The listing builds one solid part. Answer for the finished solid, in the listing's coordinates (mm). A direction names the side the tool comes from. Round coordinates to 2 decimals unless told otherwise and drop trailing zeros. Order: outer loops, then holes, each group sorted by start corner. A loop starts at its lowest first (then second) coordinate and runs counter-clockwise, first axis right, second up. Notation, with made-up numbers: M 35,73.5 L 65,73.5 A17 ccw 65,100.5 Z; hole C -14,46 d10. An arc over 180 degrees is marked long. Put each result on its own line as item: value. Start each with the question number.
1. The mould has two halves that part along X. Classify faces 1 (the face through (39, 7.3, -1)), 2 (the face through (-73, 20, 7.5)), 3 (the face through (71.993, 19.748, -40.325)): +X half, -X half, draft (parallel to the pull), parting line (faces both ways), or undercut.
2. The part is cut by section A-A (x = -49). Give the vertices of the cut face in (y, z), then the cut area to 3 significant figures.
3. Consider line 1 (Z direction, x = -65, y = 19.5); line 2 (X direction, y = 29.5, z = 23); line 3 (Y direction, x = -72.5, z = -16) (3 decimals). Determine where each line is inside the solid, lowest interval first.
4. The part is cut by section B-B (z = 5). Give the vertices of the cut face in (x, y), then the cut area to 3 significant figures.
5. The part is cut by section C-C (x = 28). Give the vertices of the cut face in (y, z).
6. Each of these flat-tipped pins is pushed along its axis until it touches: pin 1 Ø2.5 at (x, y) = (-67, 21) entering from -Z; pin 2 Ø1.5 at (x, y) = (66.5, 25) entering from +Z; pin 3 Ø2.5 at (x, y) = (68, 24) entering from -Z. Where does it stop, or does it pass through?
7. Which of the six approach directions +Z, -Z, +X, -X, +Y, -Y give full straight-line access (tool end or side, diameter ignored) to faces 4 (the face through (50.02, 7.46, 27.96)), 5 (the face through (75, 20, -1)), 6 (the face through (-73, 20, -7.5))?
from build123d import *

# Parameters (mm, degrees)
EXTRUDE_1_DEPTH     = 5
EXTRUDE_3_DEPTH     = 10
EXTRUDE_6_DEPTH     = 35
EXTRUDE_7_DEPTH     = 40
EXTRUDE_8_DEPTH     = 13
SKETCH_1_12_W       = 1
SKETCH_1_12_H       = 20
EXTRUDE_9_DEPTH     = 40
SKETCH_3_R          = 8
CUT_EXTRUDE_2_DEPTH = 5
CUT_EXTRUDE_2_DRAFT = 15
SKETCH_3_3_R        = 1.225
CUT_EXTRUDE_3_DEPTH = 5
EXTRUDE_10_DEPTH    = 7.3
EXTRUDE_11_DEPTH    = 10
SKETCH_1_17_R       = 1.225
EXTRUDE_12_DEPTH    = 35
SKETCH_4_W          = 20.2
SKETCH_4_H          = 20.2
SKETCH_4_W_2        = 15
SKETCH_4_H_2        = 15
CUT_EXTRUDE_4_DEPTH = 1
SKETCH_4_2_W        = 15
SKETCH_4_2_H        = 15
CUT_EXTRUDE_5_DEPTH = 5
SKETCH_4_4_R        = 1.225
CUT_EXTRUDE_6_DEPTH = 5
FILLET_1_R          = 2
FILLET_2_R          = 2


with BuildPart() as part:
    # Sketch 1 → Extrude 1 (new body)
    with BuildSketch(Plane(origin=(0, 0, 0), x_dir=(1, 0, 0), z_dir=(0, 1, 0))):
        with BuildLine():
            Line((75, 33.176192778), (75, -31.823807222))
            ThreePointArc((75, -31.823807222), (72.071067812, -38.894875033), (65, -41.823807222))
            Line((65, -41.823807222), (-65, -41.823807222))
            ThreePointArc((-65, -41.823807222), (-72.071067812, -38.894875033), (-75, -31.823807222))
            Line((-75, -31.823807222), (-75, 33.176192778))
            ThreePointArc((-75, 33.176192778), (-72.071067812, 40.24726059), (-65, 43.176192778))
            Line((-65, 43.176192778), (65, 43.176192778))
            ThreePointArc((65, 43.176192778), (72.071067812, 40.24726059), (75, 33.176192778))
        make_face()
    extrude(amount=EXTRUDE_1_DEPTH)

    # Sketch 1_5 → Extrude 3 (add)
    with BuildSketch(Plane(origin=(0, 0, 0), x_dir=(1, 0, 0), z_dir=(0, 1, 0))):
        Polygon((39.164167684, 31.622350466), (57.842076132, -25.396380983), (41.971862546, -30.595065501), (23.293954098, 26.423665948), align=None)
        Polygon((36.033000472, 25.440458207), (29.475846356, 23.292498736), (45.103029757, -24.413173243), (51.660183874, -22.265213771), align=None, mode=Mode.SUBTRACT)
    extrude(amount=EXTRUDE_3_DEPTH)

    # Sketch 1_7 → Extrude 6 (add)
    with BuildSketch(Plane(origin=(0, 0, 0), x_dir=(1, 0, 0), z_dir=(0, 1, 0))):
        Polygon((-15.358382401, -16.165434366), (-15.358382401, -36.823807222), (-10.358382401, -36.823807222), (-10.358382401, -22.958803378), (-10.358382401, -17.618073152), align=None)
    extrude(amount=EXTRUDE_6_DEPTH)

    # Sketch 1_8 → Extrude 7 (add)
    with BuildSketch(Plane(origin=(0, 0, 0), x_dir=(1, 0, 0), z_dir=(0, 1, 0))):
        with BuildLine():
            Line((75, -31.823807222), (75, 33.176192778))
            ThreePointArc((75, 33.176192778), (72.071067812, 40.24726059), (65, 43.176192778))
            Line((65, 43.176192778), (-65, 43.176192778))
            ThreePointArc((-65, 43.176192778), (-72.071067812, 40.24726059), (-75, 33.176192778))
            Line((-75, 33.176192778), (-75, -31.823807222))
            ThreePointArc((-75, -31.823807222), (-72.071067812, -38.894875033), (-65, -41.823807222))
            Line((-65, -41.823807222), (65, -41.823807222))
            ThreePointArc((65, -41.823807222), (72.071067812, -38.894875033), (75, -31.823807222))
        make_face()
        with BuildLine():
            Line((-60, -36.823807222), (-65, -36.823807222))
            ThreePointArc((-65, -36.823807222), (-68.535533906, -35.359341128), (-70, -31.823807222))
            Line((-70, -31.823807222), (-70, -26.823807222))
            Line((-70, -26.823807222), (-70, -10))
            Line((-70, -10), (-71, -10))
            Line((-71, -10), (-71, 10))
            Line((-71, 10), (-70, 10))
            Line((-70, 10), (-70, 28.176192778))
            Line((-70, 28.176192778), (-70, 33.176192778))
            ThreePointArc((-70, 33.176192778), (-68.535533906, 36.711726684), (-65, 38.176192778))
            Line((-65, 38.176192778), (-60, 38.176192778))
            Line((-60, 38.176192778), (60, 38.176192778))
            Line((60, 38.176192778), (65, 38.176192778))
            ThreePointArc((65, 38.176192778), (68.535533906, 36.711726684), (70, 33.176192778))
            Line((70, 33.176192778), (70, 28.176192778))
            Line((70, 28.176192778), (70, -26.823807222))
            Line((70, -26.823807222), (70, -31.823807222))
            ThreePointArc((70, -31.823807222), (68.535533906, -35.359341128), (65, -36.823807222))
            Line((65, -36.823807222), (60, -36.823807222))
            Line((60, -36.823807222), (14.702057154, -36.823807222))
            Line((14.702057154, -36.823807222), (8.624059224, -36.823807222))
            Line((8.624059224, -36.823807222), (5.895162194, -36.823807222))
            Line((5.895162194, -36.823807222), (-0.182835736, -36.823807222))
            Line((-0.182835736, -36.823807222), (-10.358382401, -36.823807222))
            Line((-10.358382401, -36.823807222), (-15.358382401, -36.823807222))
            Line((-15.358382401, -36.823807222), (-60, -36.823807222))
        make_face(mode=Mode.SUBTRACT)
    extrude(amount=EXTRUDE_7_DEPTH)

    # Sketch 1_11 → Extrude 8 (add)
    with BuildSketch(Plane(origin=(0, 0, 0), x_dir=(1, 0, 0), z_dir=(0, 1, 0))):
        Polygon((-10.358382401, -22.958803378), (-0.182835736, -36.823807222), (5.895162194, -36.823807222), (-6.056399498, -20.538839518), (-4.282789154, -19.237184284), (7.668772538, -35.522151988), (8.624059224, -36.823807222), (14.702057154, -36.823807222), (14.518227689, -36.573324733), (-3.231616409, -12.387729133), (-10.358382401, -17.618073152), align=None)
    extrude(amount=EXTRUDE_8_DEPTH)

    # Sketch 1_12 → Extrude 9 (add)
    with BuildSketch(Plane(origin=(0, 0, 0), x_dir=(1, 0, 0), z_dir=(0, 1, 0))):
        with Locations((-70.5, 0)):
            Rectangle(SKETCH_1_12_W, SKETCH_1_12_H)
    extrude(amount=EXTRUDE_9_DEPTH)


with BuildPart() as cut_extrude_2_tool:
    # Sketch 3 → Cut-Extrude 2 (with draft: the straight prism first)
    with BuildSketch(Plane.XY.offset(41.823807222)):
        with Locations((0, 20)):
            Circle(SKETCH_3_R)
    extrude(amount=-CUT_EXTRUDE_2_DEPTH)
    # Cut-Extrude 2: the draft: its side faces are tilted about the plane it starts from
    cut_extrude_2_sides = [cut_extrude_2_tool.faces().sort_by_distance(p)[0] for p in [
        (-8, 20, 39.323807222),
    ]]
    draft(cut_extrude_2_sides, Plane.XY.offset(41.823807222), CUT_EXTRUDE_2_DRAFT)


with BuildPart() as part_1:
    add(part.part)

    # Cut-Extrude 2: cut by cut_extrude_2_tool
    add(cut_extrude_2_tool.part, mode=Mode.SUBTRACT)

    # Sketch 3_3 → Cut-Extrude 3 (cut)
    with BuildSketch(Plane.XY.offset(41.823807222)):
        with Locations((56.3, 19)):
            Circle(SKETCH_3_3_R)
        with Locations((-56.3, 19)):
            Circle(SKETCH_3_3_R)
    extrude(amount=-CUT_EXTRUDE_3_DEPTH, mode=Mode.SUBTRACT)

    # Sketch 1_13 → Extrude 10 (add)
    with BuildSketch(Plane(origin=(0, 0, 0), x_dir=(1, 0, 0), z_dir=(0, 1, 0))):
        Polygon((36.033000472, 25.440458207), (29.475846356, 23.292498736), (45.103029757, -24.413173243), (51.660183874, -22.265213771), align=None)
    extrude(amount=EXTRUDE_10_DEPTH)

    # Sketch 1_16 → Extrude 11 (add)
    with BuildSketch(Plane(origin=(0, 0, 0), x_dir=(1, 0, 0), z_dir=(0, 1, 0))):
        Polygon((-6.056399498, -20.538839518), (5.895162194, -36.823807222), (8.624059224, -36.823807222), (7.668772538, -35.522151988), (-4.282789154, -19.237184284), align=None)
    extrude(amount=EXTRUDE_11_DEPTH)

    # Sketch 1_17 → Extrude 12 (add)
    # profile 1 of 4: a face of its own
    with BuildSketch(Plane(origin=(0, 0, 0), x_dir=(1, 0, 0), z_dir=(0, 1, 0))):
        with BuildLine():
            ThreePointArc((-70, -31.823807222), (-68.535533906, -35.359341128), (-65, -36.823807222))
            Line((-65, -36.823807222), (-60, -36.823807222))
            Line((-60, -36.823807222), (-60, -31.823807222))
            ThreePointArc((-60, -31.823807222), (-61.464466094, -28.288273316), (-65, -26.823807222))
            Line((-65, -26.823807222), (-70, -26.823807222))
            Line((-70, -26.823807222), (-70, -31.823807222))
        make_face()
        with Locations(Location((-65, -31.823807222, 0), (0, 0, 90))):
            Circle(SKETCH_1_17_R, mode=Mode.SUBTRACT)
    # profile 2 of 4: a face of its own
    with BuildSketch(Plane(origin=(0, 0, 0), x_dir=(1, 0, 0), z_dir=(0, 1, 0))):
        with BuildLine():
            Line((-70, 33.176192778), (-70, 28.176192778))
            Line((-70, 28.176192778), (-65, 28.176192778))
            ThreePointArc((-65, 28.176192778), (-61.464466094, 29.640658872), (-60, 33.176192778))
            Line((-60, 33.176192778), (-60, 38.176192778))
            Line((-60, 38.176192778), (-65, 38.176192778))
            ThreePointArc((-65, 38.176192778), (-68.535533906, 36.711726684), (-70, 33.176192778))
        make_face()
        with Locations(Location((-65, 33.176192778, 0), (0, 0, 90))):
            Circle(SKETCH_1_17_R, mode=Mode.SUBTRACT)
    # profile 3 of 4: a face of its own
    with BuildSketch(Plane(origin=(0, 0, 0), x_dir=(1, 0, 0), z_dir=(0, 1, 0))):
        with BuildLine():
            Line((60, -31.823807222), (60, -36.823807222))
            Line((60, -36.823807222), (65, -36.823807222))
            ThreePointArc((65, -36.823807222), (68.535533906, -35.359341128), (70, -31.823807222))
            Line((70, -31.823807222), (70, -26.823807222))
            Line((70, -26.823807222), (65, -26.823807222))
            ThreePointArc((65, -26.823807222), (61.464466094, -28.288273316), (60, -31.823807222))
        make_face()
        with Locations(Location((65, -31.823807222, 0), (0, 0, 90))):
            Circle(SKETCH_1_17_R, mode=Mode.SUBTRACT)
    # profile 4 of 4: a face of its own
    with BuildSketch(Plane(origin=(0, 0, 0), x_dir=(1, 0, 0), z_dir=(0, 1, 0))):
        with BuildLine():
            Line((65, 38.176192778), (60, 38.176192778))
            Line((60, 38.176192778), (60, 33.176192778))
            ThreePointArc((60, 33.176192778), (61.464466094, 29.640658872), (65, 28.176192778))
            Line((65, 28.176192778), (70, 28.176192778))
            Line((70, 28.176192778), (70, 33.176192778))
            ThreePointArc((70, 33.176192778), (68.535533906, 36.711726684), (65, 38.176192778))
        make_face()
        with Locations(Location((65, 33.176192778, 0), (0, 0, 90))):
            Circle(SKETCH_1_17_R, mode=Mode.SUBTRACT)
    extrude(amount=EXTRUDE_12_DEPTH)

    # Sketch 4 → Cut-Extrude 4 (cut)
    with BuildSketch(Plane(origin=(-70, 0, 0), x_dir=(0, 0, -1), z_dir=(1, 0, 0))):
        with Locations((0, 20)):
            Rectangle(SKETCH_4_W, SKETCH_4_H)
        with Locations((0, 20)):
            Rectangle(SKETCH_4_W_2, SKETCH_4_H_2, mode=Mode.SUBTRACT)
    extrude(amount=-CUT_EXTRUDE_4_DEPTH, mode=Mode.SUBTRACT)

    # Sketch 4_2 → Cut-Extrude 5 (cut)
    with BuildSketch(Plane(origin=(-70, 0, 0), x_dir=(0, 0, -1), z_dir=(1, 0, 0))):
        with Locations((0, 20)):
            Rectangle(SKETCH_4_2_W, SKETCH_4_2_H)
    extrude(amount=-CUT_EXTRUDE_5_DEPTH, mode=Mode.SUBTRACT)

    # Sketch 4_4 → Cut-Extrude 6 (cut)
    with BuildSketch(Plane(origin=(-70, 0, 0), x_dir=(0, 0, -1), z_dir=(1, 0, 0))):
        with Locations((-16, 20)):
            Circle(SKETCH_4_4_R)
        with Locations((-22, 20)):
            Circle(SKETCH_4_4_R)
        with Locations((16, 20)):
            Circle(SKETCH_4_4_R)
        with Locations((22, 20)):
            Circle(SKETCH_4_4_R)
    extrude(amount=-CUT_EXTRUDE_6_DEPTH, mode=Mode.SUBTRACT)

    # Fillet 1
    fillet_1_edges = [part_1.edges().sort_by_distance(p)[0] for p in [
        (75, 40, -0.676192778),
        (-75, 40, -0.676192778),
        (0, 40, 41.823807222),
        (72.071067812, 40, 38.894875033),
        (72.071067812, 40, -40.24726059),
        (0, 40, -43.176192778),
        (-72.071067812, 40, -40.24726059),
        (-72.071067812, 40, 38.894875033),
    ]]
    fillet(fillet_1_edges, radius=FILLET_1_R)

    # Fillet 2
    fillet_2_edges = [part_1.edges().sort_by_distance(p)[0] for p in [
        (75, 0, -0.676192778),
        (72.071067812, 0, -40.24726059),
        (0, 0, -43.176192778),
        (-72.071067812, 0, -40.24726059),
        (-75, 0, -0.676192778),
        (-72.071067812, 0, 38.894875033),
        (0, 0, 41.823807222),
        (72.071067812, 0, 38.894875033),
    ]]
    fillet(fillet_2_edges, radius=FILLET_2_R)


solid = part_1.part
Resolved:
1. face 1: undercut
1. face 2: draft
1. face 3: +X half
2. outline: M 0,-41.18 A2 ccw 2,-43.18 L 38,-43.18 A2 ccw 40,-41.18 L 40,-38.18 L 5,-38.18 L 5,36.82 L 40,36.82 L 40,39.82 A2 ccw 38,41.82 L 2,41.82 A2 ccw 0,39.82 Z
2. area: 772 mm2
3. line 1: -43.18 to -34.4, -31.95 to -28.18, 26.82 to 30.6, 33.05 to 41.82
3. line 2: -75 to -70, -15.36 to -10.36, 70 to 75
3. line 3: 0 to 18.775, 21.225 to 40
4. outline: M -75,2 A2 ccw -73,0 L 73,0 A2 ccw 75,2 L 75,38 A2 ccw 73,40 L 70,40 L 70,5 L 51.16,5 L 51.16,10 L 46,10 L 46,7.3 L 38.74,7.3 L 38.74,10 L 33.59,10 L 33.59,5 L -70,5 L -70,9.9 L -71,9.9 L -71,12.5 L -75,12.5 Z; M -75,27.5 L -71,27.5 L -71,30.1 L -70,30.1 L -70,40 L -73,40 A2 ccw -75,38 Z
4. area: 1,080 mm2
5. outline: M 0,-41.18 A2 ccw 2,-43.18 L 38,-43.18 A2 ccw 40,-41.18 L 40,-38.18 L 5,-38.18 L 5,-27.97 L 10,-27.97 L 10,-12.06 L 5,-12.06 L 5,36.82 L 40,36.82 L 40,39.82 A2 ccw 38,41.82 L 2,41.82 A2 ccw 0,39.82 Z
6. pin 1: z = -43.15
6. pin 2: z = 41.8
6. pin 3: z = -43.02
7. face 4: +Y
7. face 5: +Z, -Z, +X, +Y, -Y
7. face 6: -X
